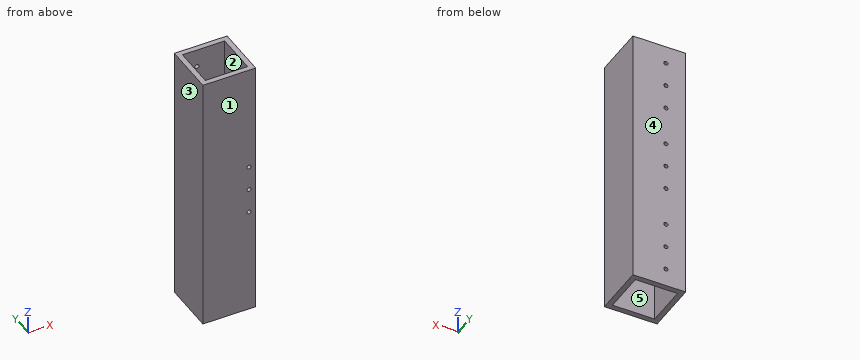
Solid Edge part; units mm, degrees
sketch "Sketch1" plane through (0, 0, 0) normal (0, 0, 1) x (1, 0, 0)
  line L0 (-33.7579, 34.8421) -> (-33.7579, -29.1579)
  line L1 (-33.7579, -29.1579) -> (30.2421, -29.1579)
  line L2 (30.2421, -29.1579) -> (30.2421, 34.8421)
  line L3 (30.2421, 34.8421) -> (-33.7579, 34.8421)
  line L4 (-41.7579, 42.8421) -> (-41.7579, -37.1579)
  line L5 (-41.7579, -37.1579) -> (38.2421, -37.1579)
  line L6 (38.2421, -37.1579) -> (38.2421, 42.8421)
  line L7 (38.2421, 42.8421) -> (-41.7579, 42.8421)
  dimension "D1" = 38.2421
  dimension "D2" = 38.2421
  dimension "D3" = 30.2421
extrude "Protrusion1" add sketch "Sketch1" along normal blind 400
hole "Hole_10" at (28.2421, -37.1579, 200) direction (0, 1, 0) diameter 6.2 depth 10
hole "Hole1" at (28.2421, -37.1579, 162.5) direction (0, 1, 0) diameter 6.2 depth 10
hole "Hole2" at (28.2421, -37.1579, 237.5) direction (0, 1, 0) diameter 6.2 depth 10
hole "Hole_13" at (-11.7579, 42.8421, 65) direction (0, -1, 0) diameter 6.2 end up to next
hole "Hole3" at (-11.7579, 42.8421, 102.5) direction (0, -1, 0) diameter 6.2 end up to next
hole "Hole4" at (-11.7579, 42.8421, 162.5) direction (0, -1, 0) diameter 6.2 end up to next
hole "Hole5" at (-11.7579, 42.8421, 200) direction (0, -1, 0) diameter 6.2 end up to next
hole "Hole6" at (-11.7579, 42.8421, 237.5) direction (0, -1, 0) diameter 6.2 end up to next
hole "Hole7" at (-11.7579, 42.8421, 297.5) direction (0, -1, 0) diameter 6.2 end up to next
hole "Hole8" at (-11.7579, 42.8421, 335) direction (0, -1, 0) diameter 6.2 end up to next
hole "Hole9" at (-11.7579, 42.8421, 372.5) direction (0, -1, 0) diameter 6.2 end up to next
hole "Hole10" at (-11.7579, 42.8421, 27.5) direction (0, -1, 0) diameter 6.2 end up to next
Source: CAD feature listing. Evaluate the final solid. Frame: model axes, mm. Face numbers are marked on the shaded views. A direction names the side the tool comes from. Give positions to 0.01 mm unless a question says otherwise; leave off trailing zeros. Order: outer loops, then holes, each group sorted by start corner. A loop starts at its lowest first (then second) coordinate and runs counter-clockwise, first axis right, second up. Notation, with made-up numbers: (-22.5, 73.25) -> (-18.5, 73.25) arc R25 ccw to (-18.5, 106.25) -> close; hole circle Ø1 at (64.5, 3). An arc over 180 degrees is marked (long way). Use a Markdown table: item, result.
Q1. Access query for the marked faces 1 and 2. Directions: +Z, -Z, +X, -X, +Y, -Y. A direction counts if a zero-diameter tool reaches every point of the face in a straight line with its end or side. Return the directions, or none.
A:
| item | result |
|---|---|
| face 1 | +Z, -Z, +X, -X, -Y |
| face 2 | +Z, -Z |
Q2. Material intervals for line 1 (Y direction, x = -29, z = 300); line 2 (X direction, y = 11, z = 197); line 3 (X direction, y = -32, z = 237), sorted ascending. Write a range as [from, to].
A:
| item | result |
|---|---|
| line 1 | [-37.16, -29.16], [34.84, 42.84] |
| line 2 | [-41.76, -33.76], [30.24, 38.24] |
| line 3 | [-41.76, 25.18], [31.3, 38.24] |
Q3. Section B-B (z = 357). Return the cut outline in (x, y).
A:
| item | result |
|---|---|
| outline | (-41.76, -37.16) -> (38.24, -37.16) -> (38.24, 42.84) -> (-41.76, 42.84) -> close; hole (-33.76, -29.16) -> (30.24, -29.16) -> (30.24, 34.84) -> (-33.76, 34.84) -> close |
Q4. First-contact query: P1, Ø5, axis at x = -11.76, z = 297.5, coming from the +Y side; P2, Ø1.2, axis at x = 30.5, z = 199, coming from the -Y side; P3, Ø3, axis at x = 23.5, y = 31.5, coming from the -Z side. Flat tips, straight axial feed; report the tip coordinate or a pass-through.
A:
| item | result |
|---|---|
| P1 | y = -29.16 |
| P2 | y = -27.16 |
| P3 | through |
Q5. Pull-direction query (Y, two-part tool) for the marked faces 3, 4 and 5; classes: +Y half, -Y half, draft (parallel to the pull), parting line (faces both ways), or undercut.
A:
| item | result |
|---|---|
| face 3 | draft |
| face 4 | +Y half |
| face 5 | undercut |
Q6. Section A-A (y = -22.5). Return the cut outline in (x, z).
A:
| item | result |
|---|---|
| outline | (-41.76, 0) -> (-33.76, 0) -> (-33.76, 400) -> (-41.76, 400) -> close; (30.24, 0) -> (38.24, 0) -> (38.24, 400) -> (30.24, 400) -> close |
